For this review, take the finished solid that the model builds, in its own axes (mm). Face numbers are marked on the shaded views. A direction names the side the tool comes from. Round coordinates to 2 decimals unless told otherwise and drop trailing zeros. Write each loop counter-clockwise with the first axis right and the second up, starting at its lowest first coordinate (ties: lowest second). Pieces come first, ordered by that corner, then holes. Notation, with made-up numbers: (9, -29) - (28, -29) arc R7 ccw to (28, -17) - close; hole circle Ø10 at (-28.5, -7). An arc over 180 degrees is marked (long way). One line per item, written item: value. Start each with the question number.
Q1. Add section D-D on y = 23.5. Write out the cut boundary in (x, z), and give its area (3 significant figures).
Q2. Clearance check with flat-ended pins moving along their axes: pin 1 Ø22.5 at (x, y) = (-35.5, 23.5) entering from -Z; pin 2 Ø12 at (x, z) = (137.5, -16) entering from +Y. State where each tip first meets the part, or that it passes through.
Q3. Tool access review of the marked faces 1 and 2: name each direction out of +Z, -Z, +X, -X, +Y, -Y from which nothing blocks a thin tool from reaching the whole face with its end or side.
Q4. Add section B-B on z = -19.76. Write out the cut boundary in (x, y).
Q5. For probe 1 along X at (y, z) = (2.45, -19.76); probe 2 along Z at (x, y) = (87.5, 1.8); probe 3 along Y at (x, z) = (-70, -25), list the stretches that pass through material, from the lowest coordinate up.
Q6. Add section C-C on x = -112. Write out the cut boundary in (y, z) (1 decimal).
```python
from build123d import *

# Parameters (mm, degrees)
A_O_CANTONEIRA_LAMINADA_1020_3_16X1_1_2_DEPTH = 350
ESBO_O4_R                                     = 4
CORTE_EXTRUS_O1_DEPTH                         = 184.107127114


with BuildPart() as part:
    # Sketch11 → Aço cantoneira laminada 1020 3-16X1-1-2(1) (new body)
    with BuildSketch(Plane(origin=(-175, 0, 0), x_dir=(0, 0, -1), z_dir=(1, 0, 0))):
        with BuildLine():
            Line((0, 0), (0, 38.1))
            Line((0, 38.1), (1.5, 38.1))
            ThreePointArc((1.5, 38.1), (3.806935874, 37.144435874), (4.7625, 34.8375))
            Line((4.7625, 34.8375), (4.7625, 6.7625))
            ThreePointArc((4.7625, 6.7625), (5.348286438, 5.348286438), (6.7625, 4.7625))
            Line((6.7625, 4.7625), (34.8375, 4.7625))
            ThreePointArc((34.8375, 4.7625), (37.144435874, 3.806935874), (38.1, 1.5))
            Line((38.1, 1.5), (38.1, 0))
            Line((38.1, 0), (0, 0))
        make_face()
    extrude(amount=A_O_CANTONEIRA_LAMINADA_1020_3_16X1_1_2_DEPTH)

    # Esboço4 → Corte-extrusão1 (cut, through all)
    with BuildSketch(Plane(origin=(0, 0, 0), x_dir=(1, 0, 0), z_dir=(0, 1, 0))):
        with Locations(Location((-87.5, 19.76, 0), (0, 0, 90))):
            Circle(ESBO_O4_R)
        with Locations(Location((87.5, 19.76, 0), (0, 0, 90))):
            Circle(ESBO_O4_R)
        with BuildLine():
            Line((-5, 12), (-5, 26.1))
            ThreePointArc((-5, 26.1), (0, 31.1), (5, 26.1))
            Line((5, 26.1), (5, 12))
            ThreePointArc((5, 12), (0, 7), (-5, 12))
        make_face()
    extrude(amount=CORTE_EXTRUS_O1_DEPTH, mode=Mode.SUBTRACT)


solid = part.part
```
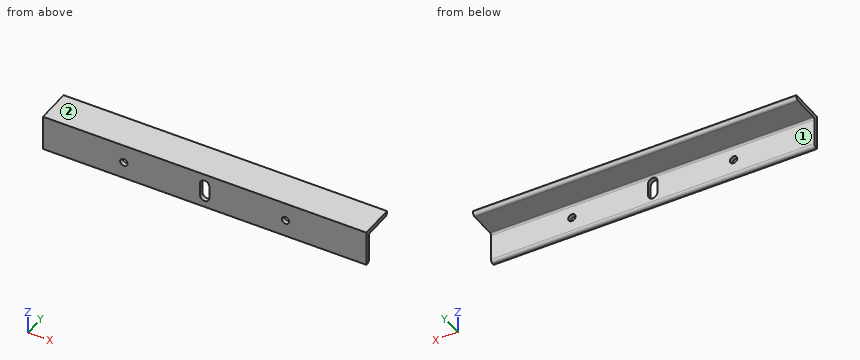
Result set:
1. outline: (-175, -4.76) - (175, -4.76) - (175, 0) - (-175, 0) - close
1. area: 1,670 mm^2
2. pin 1: stops at z = -4.76
2. pin 2: stops at y = 4.76
3. face 1: -Z, +X, -X, +Y
3. face 2: +Z, +X, -X, +Y, -Y
4. outline: (-175, 0) - (-91.5, 0) - (-91.5, 4.76) - (-175, 4.76) - close; (-83.5, 0) - (-5, 0) - (-5, 4.76) - (-83.5, 4.76) - close; (5, 0) - (83.5, 0) - (83.5, 4.76) - (5, 4.76) - close; (91.5, 0) - (175, 0) - (175, 4.76) - (91.5, 4.76) - close
5. probe 1: x = -175 to -91.5, -83.5 to -5, 5 to 83.5, 91.5 to 175
5. probe 2: z = -38.09 to -23.76, -15.76 to 0
5. probe 3: y = 0 to 4.76
6. outline: (0, -38.1) - (1.5, -38.1) arc R3.3 ccw to (4.8, -34.8) - (4.8, -6.8) arc R2 cw to (6.8, -4.8) - (34.8, -4.8) arc R3.3 ccw to (38.1, -1.5) - (38.1, 0) - (0, 0) - close
